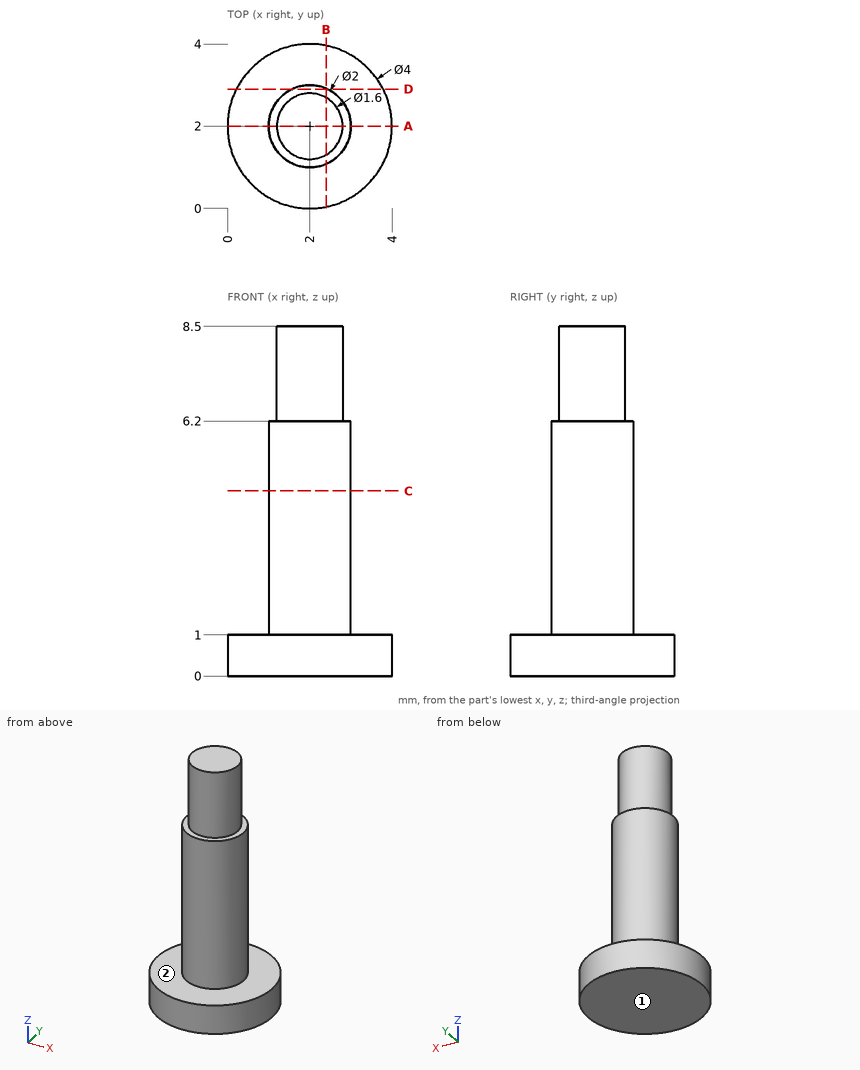
Part print with two shaded views. Sizes in mm from the minimum x, y, z corner. A direction names the side the tool comes from. Round coordinates to 2 decimals unless told otherwise and drop trailing zeros. Write each loop counter-clockwise with the first axis right and the second up, starting at its lowest first coordinate (ties: lowest second). Pieces come first, ordered by that corner, then holes. Notation, with made-up numbers: (85.5, 41.25) - (100.5, 41.25) arc R20 ccw to (100.5, 69.25) - close; hole circle Ø6 at (-31, 4.25). An arc over 180 degrees is marked (long way). Use CSV: the item, a comma, the result in double quotes.
Item 1: Slice it at B-B, the plane x = 2.4. Write the cut outline in (y, z).
Results list:
outline,"(0.04, 0) - (3.96, 0) - (3.96, 1) - (2.92, 1) - (2.92, 6.2) - (2.69, 6.2) - (2.69, 8.5) - (1.31, 8.5) - (1.31, 6.2) - (1.08, 6.2) - (1.08, 1) - (0.04, 1) - close"
Item 2: Slice it at D-D, the plane y = 2.9. Write the cut outline in (x, z).
Results list:
outline,"(0.21, 0) - (3.79, 0) - (3.79, 1) - (2.44, 1) - (2.44, 6.2) - (1.56, 6.2) - (1.56, 1) - (0.21, 1) - close"
Item 3: Wall check: L1, parallel to Z at x = 0.8, y = 1.05; L2, parallel to Z at x = 2.9, y = 2; L3, parallel to Y at x = 2, z = 6. Give the ranges that are in metal, low to high.
Results list:
L1,"z = 0 to 1"
L2,"z = 0 to 6.2"
L3,"y = 1 to 3"
Item 4: Slice it at C-C, the plane z = 4.5. Write the cut outline in (x, y), then the cut area to 3 significant figures.
Results list:
outline,"circle Ø2 at (2, 2)"
area,"3.14 mm²"
Item 5: Slice it at A-A, the plane y = 2. Write the cut outline in (x, z).
Results list:
outline,"(0, 0) - (4, 0) - (4, 1) - (3, 1) - (3, 6.2) - (2.8, 6.2) - (2.8, 8.5) - (1.2, 8.5) - (1.2, 6.2) - (1, 6.2) - (1, 1) - (0, 1) - close"
Item 6: Tool access for the marked faces 1 and 2: list every direction of +Z, -Z, +X, -X, +Y, -Y with a clear straight run to the whole face (end or side of a thin tool).
Results list:
face 1,"-Z, +X, -X, +Y, -Y"
face 2,"+Z"
